from build123d import *

# Parameters (mm, degrees)
BASPROSKE_W                                    = 7
BASPROSKE_H                                    = 22
TOOTHCUT_DEPTH                                 = 32.890437438
TEETHCUTS_COUNT                                = 20
TEETHCUTS_ANGLE                                = 342
BORSKE_R                                       = 3.5
BORE_DEPTH                                     = 50.0000508
FRAISAGE_POUR_VIS_T_TE_FRAIS_E_M21_D           = 2.4
FRAISAGE_POUR_VIS_T_TE_FRAIS_E_M21_CSINK_D     = 4.4
FRAISAGE_POUR_VIS_T_TE_FRAIS_E_M21_CSINK_ANGLE = 90
R_P_TITION_CIRCULAIRE1_COUNT                   = 4


with BuildPart() as part:
    # BasProSke → Base-Revolve (revolve)
    with BuildSketch(Plane(origin=(0, 0, 0), x_dir=(1, 0, 0), z_dir=(0, 1, 0)), mode=Mode.PRIVATE) as base_revolve_sk:
        with Locations((3.5, 11)):
            Rectangle(BASPROSKE_W, BASPROSKE_H)
    revolve(base_revolve_sk.sketch.rotate(Axis((-10, 0, 0), (1, 0, 0)), 180), axis=Axis((-10, 0, 0), (1, 0, 0)))

    # TooCutSke → ToothCut (cut, through all)
    with BuildSketch(Plane(origin=(0, 0, 0), x_dir=(0, 0, -1), z_dir=(1, 0, 0))):
        with BuildLine():
            ThreePointArc((0.986171591, 17.471189616), (0, 17.499), (-0.986171591, 17.471189616))
            ThreePointArc((-0.986171591, 17.471189616), (-1.626916196, 19.798789858), (-2.932850173, 21.829260982))
            ThreePointArc((-2.932850173, 21.829260982), (0, 22.0254), (2.932850173, 21.829260982))
            ThreePointArc((2.932850173, 21.829260982), (1.626916196, 19.798789858), (0.986171591, 17.471189616))
        make_face()
    toothcut = extrude(amount=TOOTHCUT_DEPTH, mode=Mode.SUBTRACT)

    # TeethCuts: ToothCut ×20 about axis
    teethcuts_axis = Axis((-10, 0, 0), (1, 0, 0))
    for i in range(1, TEETHCUTS_COUNT):
        add(toothcut.rotate(teethcuts_axis, i * TEETHCUTS_ANGLE / (TEETHCUTS_COUNT - 1)), mode=Mode.SUBTRACT)

    # BorSke → Bore (cut, symmetric)
    with BuildSketch(Plane(origin=(0, 0, 0), x_dir=(0, 0, -1), z_dir=(1, 0, 0))):
        with Locations(Location((0, 0, 0), (0, 0, 180))):
            Circle(BORSKE_R)
    extrude(amount=BORE_DEPTH, both=True, mode=Mode.SUBTRACT)

    # Fraisage pour vis à tête fraisée M21 (through all)
    with Locations(Plane(origin=(7, 0, 0), x_dir=(0, 0, -1), z_dir=(1, 0, 0))):
        with Locations((1.298006129, 7.893996459)):
            fraisage_pour_vis_t_te_frais_e_m21 = CounterSinkHole(FRAISAGE_POUR_VIS_T_TE_FRAIS_E_M21_D / 2, FRAISAGE_POUR_VIS_T_TE_FRAIS_E_M21_CSINK_D / 2, counter_sink_angle=FRAISAGE_POUR_VIS_T_TE_FRAIS_E_M21_CSINK_ANGLE)

    # Répétition circulaire1: Fraisage pour vis à tête fraisée M21 ×4 about axis
    r_p_tition_circulaire1_axis = Axis((0, 0, 0), (1, 0, 0))
    for i in range(1, R_P_TITION_CIRCULAIRE1_COUNT):
        add(fraisage_pour_vis_t_te_frais_e_m21.rotate(r_p_tition_circulaire1_axis, i * 360 / R_P_TITION_CIRCULAIRE1_COUNT), mode=Mode.SUBTRACT)


solid = part.part
Source: CAD feature listing. Evaluate the final solid. Frame: model axes, mm. A direction names the side the tool comes from. Coordinates: 2 decimals unless noted, no trailing zeros. Loops run counter-clockwise (first coordinate to the right, second up) from the corner with the lowest first, then second, coordinate; pieces in that order, holes last. Notation, with made-up numbers: M -4,-22 L 8,-22 A20 cw 8,-10 Z; hole C -17,37.5 d9. An arc over 180 degrees is marked long. Answer in a Markdown table with one row per item.
Q1. First-contact query: pin 1 (4 mm diameter, centred on x = 2.5, z = 10.5, fed in from -Y); pin 2 (12 mm diameter, centred on y = 17, z = -10.5, fed in from -X); pin 3 (4 mm diameter, centred on x = 2.5, z = -8, fed in from +Y). Flat tips, straight axial feed; report the tip coordinate or a pass-through.
Answers below:
| item | result |
|---|---|
| pin 1 | stops at y = -19.84 |
| pin 2 | stops at x = 0 |
| pin 3 | stops at y = 19.84 |
Q2. Section D-D on z = -12. Return the cut outline in (x, y), plus the area to 3 significant figures.
Answers below:
| item | result |
|---|---|
| outline | M 0,-14.42 L 7,-14.42 L 7,14.42 L 0,14.42 Z |
| area | 202 mm^2 |
Q3. Section A-A on z = 18.5. Return the cut outline in (x, y).
Answers below:
| item | result |
|---|---|
| outline | M 0,-10.49 L 7,-10.49 L 7,-7.83 L 0,-7.83 Z; M 0,-4.62 L 7,-4.62 L 7,-1.18 L 0,-1.18 Z; M 0,1.18 L 7,1.18 L 7,4.62 L 0,4.62 Z; M 0,7.83 L 7,7.83 L 7,10.49 L 0,10.49 Z |
Q4. Draft query along Y for faces 1 (the cylindrical face through (3.451, -7.678, -18.341)), 2 (the cylindrical face through (3.45, -15.07, 12.97)), 3 (the cylindrical face through (3.5, 17.5, 0)). Return one class per face: pulls with the +Y half, pulls with the -Y half, needs draft (parallel to the pull), parting line crosses it, or undercut.
Answers below:
| item | result |
|---|---|
| face 1 | undercut |
| face 2 | pulls with the -Y half |
| face 3 | pulls with the +Y half |
Q5. Ray query, probe 1 along Z at (x, y) = (5.75, 15); probe 2 along Z at (x, y) = (2, 15.5); probe 3 along Y at (x, z) = (4.25, -2). Return the intervals inside material, ascending. Write a range as from..to.
Answers below:
| item | result |
|---|---|
| probe 1 | z = -15.89..-12.85, -9.62..9.62, 12.85..15.89 |
| probe 2 | z = -15.61..-13.84, -9.86..9.86, 13.84..15.61 |
| probe 3 | y = -20.53..-2.87, 2.87..6.92, 8.87..20.53 |
Q6. Set-up query: faces 4 (the cylindrical face through (3.451, -4.576, -19.284)), 5 (the cylindrical face through (3.549, 21.728, -3.449)), 6 (the cylindrical face through (3.451, -18.341, 7.678)), 7 (the cylindrical face through (3.549, 3.449, 21.728)), 8 (the cylindrical face through (3.451, 15.037, 12.911)). Return all of +Z, -Z, +X, -X, +Y, -Y with unobstructed straight access to the full face (end or side cutting, diameter ignored); none if empty.
Answers below:
| item | result |
|---|---|
| face 4 | +X, -X |
| face 5 | -Z, +X, -X, +Y |
| face 6 | +X, -X, -Y |
| face 7 | +Z, +X, -X, +Y |
| face 8 | +X, -X, +Y |
Q7. Section B-B on z = 1.5. State how many separate pieces and enclosed holes the cut face has, plus the area to 3 significant figures.
Answers below:
| item | result |
|---|---|
| separate pieces | 3 |
| enclosed holes | 0 |
| area | 211 mm^2 |
